```python
from build123d import *

# Parameters (mm, degrees)
F1_DEPTH = 1.5
F2_W     = 15.637528
F2_H     = 1.5
F3_DEPTH = 12


with BuildPart() as f1:
    # F0 (on Top) → F1 (new body)
    with BuildSketch(Plane.XY):
        Polygon((-5.091527, 12.161472), (-29.960176, 12.161472), (-29.960176, 7.661472), (-19.016238, 4.523348), (-15.758272, -6.838528), (9.13308, -6.838528), (9.13308, 15.466857), (6.43572, 15.466857), align=None)
    extrude(amount=F1_DEPTH)

    # F2 (on face) → F3 (join)
    with BuildSketch(Plane.XY.offset(1.5)):
        Polygon((-29.960176, 9.061472), (-29.960176, 7.661472), (-19.016238, 4.523348), (-15.758272, -6.838528), (9.13308, -6.838528), (9.13308, -5.338528), (-14.322648, -5.338528), (-14.322648, 9.061472), align=None)
        with Locations((-22.141412, 11.411472)):
            Rectangle(F2_W, F2_H)
        Polygon((-10.322648, 10.661472), (9.13308, 10.661472), (9.13308, 15.466857), (6.43572, 15.466857), (-5.091527, 12.161472), align=None)
    extrude(amount=F3_DEPTH)


solid = f1.part
```
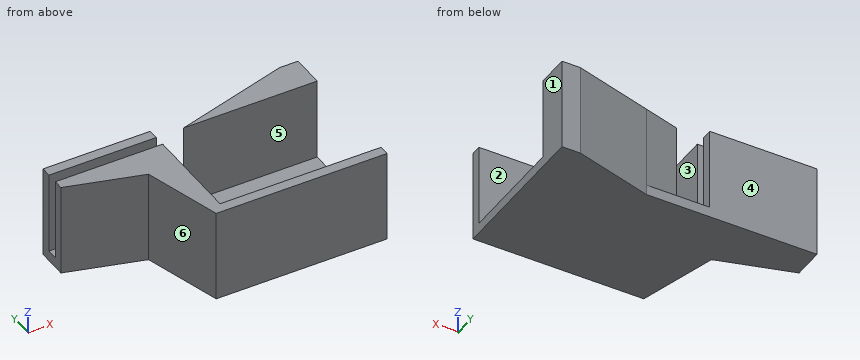
The listing builds one solid part. Answer for the finished solid, in the listing's coordinates (mm). Face numbers are marked on the shaded views. A direction names the side the tool comes from. Coordinates: 2 decimals unless noted, no trailing zeros. Write each loop counter-clockwise with the first axis right and the second up, starting at its lowest first coordinate (ties: lowest second). Pieces come first, ordered by that corner, then holes. Notation, with made-up numbers: (-37, -4.5) - (13, -4.5) arc R15 ccw to (13, 22.5) - close; hole circle Ø2 at (77.5, -35). An arc over 180 degrees is marked (long way). Return JSON: item names as keys, results as strings. Group by question number.
1. Given pin 1 (10 mm diameter, centred on x = -3, y = -2, fed in from -Z); pin 2 (6 mm diameter, centred on x = -7, z = 9.5, fed in from +Y); pin 3 (1 mm diameter, centred on y = 1, z = 8.5, fed in from +X); pin 4 (3.5 mm diameter, centred on x = -22, z = 6, fed in from +Y), each flat-ended and moving along its own axis, determine where each tip first touches the part or whether it passes through.
2. Straight lines are drawn through the part: L1, parallel to Z at x = -9.5, y = 1.75; L2, parallel to Y at x = -24.5, z = 8.5; L3, parallel to X at y = 8.5, z = 8.5. For each, find the intervals that lie inside material, in ascending order.
3. Determine the mould class of the marked faces 4, 5 and 6 for opening direction Y: released by +Y, released by -Y, zero draft, split by the parting line, or undercut.
4. A cutting plane is placed at C-C, the plane y = -3.5. Determine the outline of the cut face in (x, z).
5. A cutting plane is placed at D-D, the plane x = 0.5. Determine the outline of the cut face in (y, z).
6. A cutting plane is placed at A-A, the plane z = 5.5. Determine the outline of the cut face in (x, y), plus the area to 3 significant figures.
7. A cutting plane is placed at B-B, the plane x = -4. Determine the outline of the cut face in (y, z), plus the area to 3 significant figures.
8. Which of the six approach directions +Z, -Z, +X, -X, +Y, -Y give full straight-line access (tool end or side, diameter ignored) to the marked faces 1, 2 and 3?
Ans:
{
 "1": {"pin 1": "z = 0", "pin 2": "y = 12.47", "pin 3": "x = -14.32", "pin 4": "y = 12.16"},
 "2": {"L1": "0 to 1.5", "L2": "6.1 to 9.06, 10.66 to 12.16", "L3": "-29.96 to -14.32"},
 "3": {"face 4": "released by +Y", "face 5": "undercut", "face 6": "released by -Y"},
 "4": {"outline": "(-16.72, 0) - (9.13, 0) - (9.13, 1.5) - (-14.32, 1.5) - (-14.32, 13.5) - (-16.72, 13.5) - close"},
 "5": {"outline": "(-6.84, 0) - (13.76, 0) - (13.76, 13.5) - (10.66, 13.5) - (10.66, 1.5) - (-5.34, 1.5) - (-5.34, 13.5) - (-6.84, 13.5) - close"},
 "6": {"outline": "(-29.96, 7.66) - (-19.02, 4.52) - (-15.76, -6.84) - (9.13, -6.84) - (9.13, -5.34) - (-14.32, -5.34) - (-14.32, 9.06) - (-29.96, 9.06) - close; (-29.96, 10.66) - (-14.32, 10.66) - (-14.32, 12.16) - (-29.96, 12.16) - close; (-10.32, 10.66) - (9.13, 10.66) - (9.13, 15.47) - (6.44, 15.47) - close", "area": "200 mm²"},
 "7": {"outline": "(-6.84, 0) - (12.47, 0) - (12.47, 13.5) - (10.66, 13.5) - (10.66, 1.5) - (-5.34, 1.5) - (-5.34, 13.5) - (-6.84, 13.5) - close", "area": "68.7 mm²"},
 "8": {"face 1": "+Z, -Z, +X, +Y, -Y", "face 2": "+Z, +X", "face 3": "+Z, +X, +Y"}
}
